For this review, take the finished solid that the model builds, in its own axes (mm). Face numbers are marked on the shaded views. Round coordinates to 2 decimals unless told otherwise and drop trailing zeros. Write each loop counter-clockwise with the first axis right and the second up, starting at its lowest first coordinate (ties: lowest second). Pieces come first, ordered by that corner, then holes. Notation, with made-up numbers: (10.5, -36) -> (68.5, -36) arc R25 cw to (68.5, -16) -> close; hole circle Ø2 at (34.5, 73.5). An arc over 180 degrees is marked (long way). Answer as CSV lines item,"result". Start each with the question number.
Item 1: Take a section at B-B on y = 24.25. Give the boundary of the cut face in (x, z) (3 decimals).
Item 2: Wall thickness on probe 1 along X at (y, z) = (-24.25, 0.75); probe 2 along Y at (x, z) = (-15, 1.2); probe 3 along Y at (x, z) = (-16, 1.9): over which ranges is each line inside the solid? List them lowest first. Write a range as from..to.
Item 3: Take a section at D-D on y = -15. Give the boundary of the cut face in (x, z), then the cut area to 3 significant figures.
Item 4: Take a section at C-C on z = 2.15. Give the boundary of the cut face in (x, y).
Item 5: Take a section at A-A on x = 20.5. Give the boundary of the cut face in (y, z).
Item 6: For pin 1 Ø6 at (x, y) = (-13.5, 24) entering from +Z; pin 2 Ø4 at (x, y) = (-15, 24.25) entering from +Z; pin 3 Ø2 at (y, z) = (16, 1.5) entering from -X, all flat-tipped, find the tip position at first contact; note any pin that passes through.
Item 7: Mouldability with a two-part tool opening along Z and no side actions: class the marked faces 1 and 2 as +Z half, -Z half, draft (parallel to the pull), parting line (faces both ways), or undercut.
```python
from build123d import *

# Parameters (mm, degrees)
SKIZZE1_R                       = 1.65
AUFSATZ_LINEAR_AUSTRAGEN1_DEPTH = 5
SKIZZE2_R                       = 3.65
SCHNITT_LINEAR_AUSTRAGEN1_DEPTH = 4
VERRUNDUNG10_R                  = 1


with BuildPart() as part:
    # Skizze1 → Aufsatz-Linear austragen1 (new body)
    with BuildSketch(Plane.XY):
        with BuildLine():
            Line((25.22, 27.5), (17.320508076, 27.5))
            ThreePointArc((17.320508076, 27.5), (-32.5, 0), (17.320508076, -27.5))
            Line((17.320508076, -27.5), (25.22, -27.5))
            Line((25.22, -27.5), (25.22, 27.5))
        make_face()
        with Locations((20.5, -24.25)):
            Circle(SKIZZE1_R, mode=Mode.SUBTRACT)
        with Locations((20.5, 24.25)):
            Circle(SKIZZE1_R, mode=Mode.SUBTRACT)
        with Locations((-15, -24.25)):
            Circle(SKIZZE1_R, mode=Mode.SUBTRACT)
        with Locations((-15, 24.25)):
            Circle(SKIZZE1_R, mode=Mode.SUBTRACT)
    extrude(amount=AUFSATZ_LINEAR_AUSTRAGEN1_DEPTH)

    # Skizze2 → Schnitt-Linear austragen1 (cut)
    with BuildSketch(Plane.XY.offset(5)):
        with Locations((-15, 24.25)):
            Circle(SKIZZE2_R)
        with Locations((20.5, 24.25)):
            Circle(SKIZZE2_R)
        with Locations((20.5, -24.25)):
            Circle(SKIZZE2_R)
        with Locations(Location((-15, -24.25, 0), (0, 0, 180))):
            Circle(SKIZZE2_R)
    extrude(amount=-SCHNITT_LINEAR_AUSTRAGEN1_DEPTH, mode=Mode.SUBTRACT)

    # Verrundung10
    # the kernel refuses this fillet: 1 mm, written as the material it takes off along each edge
    with BuildSketch(Plane(origin=(25.22, -30, 5), x_dir=(-1, 0, 0), z_dir=(0, 1, 0))) as verrundung10_piece_1:
        with BuildLine():
            CenterArc((VERRUNDUNG10_R, -VERRUNDUNG10_R), VERRUNDUNG10_R, 90, 90)
            Line((0, -VERRUNDUNG10_R), (0, 0))
            Line((0, 0), (VERRUNDUNG10_R, 0))
        make_face()
    extrude(amount=60, mode=Mode.SUBTRACT)
    with BuildSketch(Plane(origin=(20.5, 24.25, 5), x_dir=(0.0031415874858533787, 0.9999950652018582, 0), z_dir=(-0.9999950652018582, 0.0031415874858533787, 0))) as verrundung10_piece_2:
        with BuildLine():
            CenterArc((3.65 + VERRUNDUNG10_R, VERRUNDUNG10_R), VERRUNDUNG10_R, 180, 90)
            Line((3.65 + VERRUNDUNG10_R, 0), (3.65, 0))
            Line((3.65, 0), (3.65, VERRUNDUNG10_R))
        make_face()
    revolve(axis=Axis((20.5, 24.25, 5), (0, 0, -1)), revolution_arc=359.64, mode=Mode.SUBTRACT)
    with BuildSketch(Plane(origin=(20.5, -24.25, 5), x_dir=(-0.0031415874859059387, -0.999995065201858, 0), z_dir=(0.999995065201858, -0.0031415874859059387, 0))) as verrundung10_piece_3:
        with BuildLine():
            CenterArc((3.65 + VERRUNDUNG10_R, VERRUNDUNG10_R), VERRUNDUNG10_R, 180, 90)
            Line((3.65 + VERRUNDUNG10_R, 0), (3.65, 0))
            Line((3.65, 0), (3.65, VERRUNDUNG10_R))
        make_face()
    revolve(axis=Axis((20.5, -24.25, 5), (0, 0, -1)), revolution_arc=359.64, mode=Mode.SUBTRACT)
    with BuildSketch(Plane(origin=(-15, -24.25, 5), x_dir=(-1, 0, 0), z_dir=(0, 1, 0))) as verrundung10_piece_4:
        with BuildLine():
            CenterArc((3.65 + VERRUNDUNG10_R, -VERRUNDUNG10_R), VERRUNDUNG10_R, 90, 90)
            Line((3.65, -VERRUNDUNG10_R), (3.65, 0))
            Line((3.65, 0), (3.65 + VERRUNDUNG10_R, 0))
        make_face()
    revolve(axis=Axis((-15, -24.25, 5), (0, 0, 1)), mode=Mode.SUBTRACT)
    with BuildSketch(Plane(origin=(-15, 24.25, 5), x_dir=(1, 0, 0), z_dir=(0, -1, 0))) as verrundung10_piece_5:
        with BuildLine():
            CenterArc((3.65 + VERRUNDUNG10_R, -VERRUNDUNG10_R), VERRUNDUNG10_R, 90, 90)
            Line((3.65, -VERRUNDUNG10_R), (3.65, 0))
            Line((3.65, 0), (3.65 + VERRUNDUNG10_R, 0))
        make_face()
    revolve(axis=Axis((-15, 24.25, 5), (0, 0, 1)), mode=Mode.SUBTRACT)


solid = part.part
```
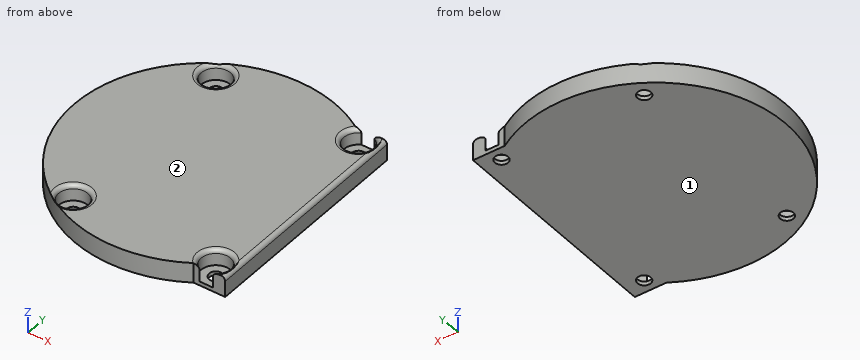
Output values:
1,outline,"(-21.638, 0) -> (-16.65, 0) -> (-16.65, 1) -> (-18.65, 1) -> (-18.65, 4) arc R1 ccw to (-19.65, 5) -> (-21.638, 5) -> close; (-13.35, 0) -> (18.85, 0) -> (18.85, 1) -> (16.85, 1) -> (16.85, 4) arc R1 ccw to (15.85, 5) -> (-10.35, 5) arc R1 ccw to (-11.35, 4) -> (-11.35, 1) -> (-13.35, 1) -> close; (22.15, 0) -> (25.22, 0) -> (25.22, 4) arc R1 ccw to (24.685, 4.885) arc R1 ccw to (24.15, 4) -> (24.15, 1) -> (22.15, 1) -> close"
2,probe 1,"x = -21.64..-16.65, -13.35..18.85, 22.15..25.22"
2,probe 2,"y = -28.83..-27.9, -20.6..20.6, 27.9..28.83"
2,probe 3,"y = -28.29..-27.76, -20.74..20.74, 27.76..28.29"
3,outline,"(-28.83, 0) -> (25.22, 0) -> (25.22, 4) arc R1 ccw to (24.22, 5) -> (-28.83, 5) -> close"
3,area,"270 mm^2"
4,outline,"(17.32, -27.5) -> (18.84, -27.5) arc R3.65 cw (long way) to (22.16, -27.5) -> (25.22, -27.5) -> (25.22, 27.5) -> (22.16, 27.5) arc R3.65 cw (long way) to (18.84, 27.5) -> (17.32, 27.5) arc R32.5 ccw (long way) to start; hole circle Ø7.3 at (-15, -24.25); hole circle Ø7.3 at (-15, 24.25)"
5,outline,"(-27.5, 0) -> (-25.9, 0) -> (-25.9, 1) -> (-27.5, 1) -> close; (-22.6, 0) -> (22.6, 0) -> (22.6, 1) -> (20.6, 1) -> (20.6, 4) arc R1 ccw to (19.6, 5) -> (-19.6, 5) arc R1 ccw to (-20.6, 4) -> (-20.6, 1) -> (-22.6, 1) -> close; (25.9, 0) -> (27.5, 0) -> (27.5, 1) -> (25.9, 1) -> close"
6,pin 1,"stops at z = 4.99"
6,pin 2,"stops at z = 1"
6,pin 3,"stops at x = -28.83"
7,face 1,"-Z half"
7,face 2,"+Z half"
